```python
from build123d import *

# Parameters (mm, degrees)
MODEL_W             = 40
MODEL_H             = 110
MODEL_R             = 3
MODEL_R_2           = 1
MODEL_W_2           = 3
MODEL_H_2           = 37
MODEL_W_3           = 24.4
MODEL_H_3           = 27.5
MODEL_W_4           = 2.5
MODEL_H_4           = 10
BOSS_EXTRUDE1_DEPTH = 5
FILLET1_R           = 2


with BuildPart() as part:
    # Model → Boss-Extrude1 (new body)
    with BuildSketch(Plane.XY):
        with Locations((20, 55)):
            Rectangle(MODEL_W, MODEL_H)
        with Locations((34, 6)):
            Circle(MODEL_R, mode=Mode.SUBTRACT)
        with Locations((6, 6)):
            Circle(MODEL_R, mode=Mode.SUBTRACT)
        with Locations((20, 6)):
            Circle(MODEL_R_2, mode=Mode.SUBTRACT)
        with Locations((20, 47)):
            Circle(MODEL_R_2, mode=Mode.SUBTRACT)
        with Locations((20, 26.5)):
            Rectangle(MODEL_W_2, MODEL_H_2, mode=Mode.SUBTRACT)
        with Locations((20, 89)):
            Rectangle(MODEL_W_3, MODEL_H_3, mode=Mode.SUBTRACT)
        with Locations((11.11, 60.25)):
            Rectangle(MODEL_W_4, MODEL_H_4, mode=Mode.SUBTRACT)
        with Locations((28.89, 60.25)):
            Rectangle(MODEL_W_4, MODEL_H_4, mode=Mode.SUBTRACT)
    extrude(amount=BOSS_EXTRUDE1_DEPTH)

    # Fillet1
    fillet1_edges = [part.edges().sort_by_distance(p)[0] for p in [
        (0, 0, 2.5),
        (0, 110, 2.5),
        (40, 110, 2.5),
        (40, 0, 2.5),
    ]]
    fillet(fillet1_edges, radius=FILLET1_R)


solid = part.part
```
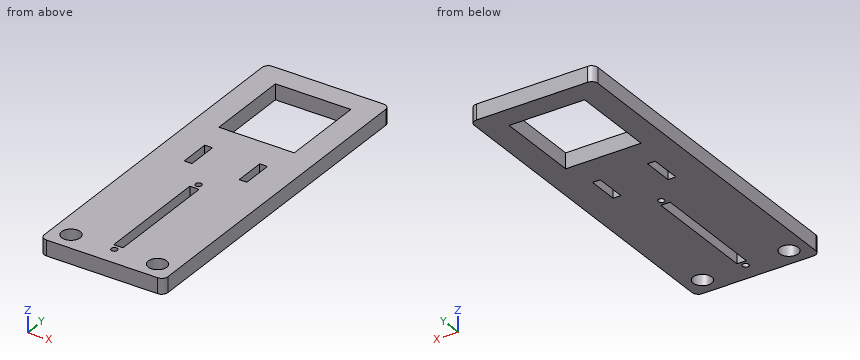
The listing builds one solid part. Answer for the finished solid, in the listing's coordinates (mm). Round coordinates to 2 decimals unless told otherwise and drop trailing zeros. Loops run counter-clockwise (first coordinate to the right, second up) from the corner with the lowest first, then second, coordinate; pieces in that order, holes last.
1) A cutting plane is placed at D-D on y = 47. Determine the outline of the cut face in (x, z).
Outcome:
outline: (0, 0) - (19, 0) - (19, 5) - (0, 5) - close; (21, 0) - (40, 0) - (40, 5) - (21, 5) - close
2) A cutting plane is placed at A-A on y = 6. Determine the outline of the cut face in (x, z), plus the area to 3 significant figures.
Outcome:
outline: (0, 0) - (3, 0) - (3, 5) - (0, 5) - close; (9, 0) - (19, 0) - (19, 5) - (9, 5) - close; (21, 0) - (31, 0) - (31, 5) - (21, 5) - close; (37, 0) - (40, 0) - (40, 5) - (37, 5) - close
area: 130 mm2
3) Consider line 1 (X direction, y = 56, z = 1.05); line 2 (X direction, y = 90.5, z = 1.3); line 3 (X direction, y = 38.5, z = 0.65). Determine where each line is inside the solid, lowest interval first.
Outcome:
line 1: x = 0 to 9.86, 12.36 to 27.64, 30.14 to 40
line 2: x = 0 to 7.8, 32.2 to 40
line 3: x = 0 to 18.5, 21.5 to 40
4) A cutting plane is placed at C-C on x = 20. Determine the outline of the cut face in (y, z), plus the area to 4 significant figures.
Outcome:
outline: (0, 0) - (5, 0) - (5, 5) - (0, 5) - close; (7, 0) - (8, 0) - (8, 5) - (7, 5) - close; (45, 0) - (46, 0) - (46, 5) - (45, 5) - close; (48, 0) - (75.25, 0) - (75.25, 5) - (48, 5) - close; (102.75, 0) - (110, 0) - (110, 5) - (102.75, 5) - close
area: 207.5 mm2
5) A cutting plane is placed at B-B on x = 6. Determine the outline of the cut face in (y, z).
Outcome:
outline: (0, 0) - (3, 0) - (3, 5) - (0, 5) - close; (9, 0) - (110, 0) - (110, 5) - (9, 5) - close
